Can you work these out from the model? Positions are in its coordinate system, mm. A direction names the side the tool comes from. Give positions to 0.01 mm unless a question says otherwise; leave off trailing zeros. Order: outer loops, then holes, each group sorted by start corner. A loop starts at its lowest first (then second) coordinate and runs counter-clockwise, first axis right, second up. Notation, with made-up numbers: (68, -11) - (103, -11) arc R8 ccw to (103, 2) - close; hole circle Ø8 at (48.5, 28). An arc over 180 degrees is marked (long way). Return JSON: item names as keys, results as strings.
```python
from build123d import *

# Parameters (mm, degrees)
SKETCH1_R           = 1.606483672
SKETCH1_R_2         = 1.474719506
BOSS_EXTRUDE1_DEPTH = 1
BOSS_EXTRUDE2_START = -2.5
SKETCH1_3_R         = 1.474719506
SKETCH1_3_R_2       = 1.606483672
BOSS_EXTRUDE2_DEPTH = 2.5


with BuildPart() as part:
    # Sketch1 → Boss-Extrude1 (new body)
    with BuildSketch(Plane(origin=(0, 0, 0), x_dir=(1, 0, 0), z_dir=(0, 1, 0))):
        with BuildLine():
            ThreePointArc((-516.919741048, 9.197616983), (-515.869047512, 9.418519621), (-514.947021866, 8.868407277))
            Line((-514.947021866, 8.868407277), (-509.711678857, 40.240087315))
            ThreePointArc((-509.711678857, 40.240087315), (-510.755516658, 40.060266208), (-511.684398038, 40.569297021))
            Line((-511.684398038, 40.569297021), (-516.919741048, 9.197616983))
        make_face()
        with Locations((-510.491081649, 41.644836785)):
            Circle(SKETCH1_R)
        with Locations((-516.1117935, 7.963915892)):
            Circle(SKETCH1_R_2)
    extrude(amount=BOSS_EXTRUDE1_DEPTH)

    # Sketch1_3 → Boss-Extrude2 (add)
    with BuildSketch(Plane(origin=(0, 0, 0), x_dir=(1, 0, 0), z_dir=(0, 1, 0)).offset(BOSS_EXTRUDE2_START)):
        with Locations(Location((-516.1117935, 7.963915892, 0), (0, 0, 123.220682047))):
            Circle(SKETCH1_3_R)
        with Locations(Location((-510.491081649, 41.644836785, 0), (0, 0, 222.028435657))):
            Circle(SKETCH1_3_R_2)
    extrude(amount=BOSS_EXTRUDE2_DEPTH)


solid = part.part
```
1. On a 3-axis mill with a long thin cutter (end or side, diameter ignored), from which of +Z, -Z, +X, -X, +Y, -Y can I reach the whole of each face in a straight line? I mean faces 4 (the face through (-510.199, -0.774, -43.224)), 5 (the face through (-510, -2.5, -42)). Say none if no direction works.
Checks:
{"face 4": "-Y", "face 5": "+Z, -Z, +X, -X, -Y"}
2. Suppose I cut it at C-C (z = -41). List the corners of the cut face in (x, y) for me.
Checks:
{"outline": "(-511.96, -2.5) - (-509.02, -2.5) - (-509.02, 1) - (-511.96, 1) - close"}
3. Thinking about a two-plate mould opening in Y: for faces 1 (the face through (-513, 1, -25)), 2 (the face through (-516, -2.5, -8)), 3 (the face through (-514.265, 0.493, -25.103)), which applies, +Y half, -Y half, draft (parallel to the pull), parting line (faces both ways), or undercut?
Checks:
{"face 1": "+Y half", "face 2": "-Y half", "face 3": "draft"}
4. Suppose I cut it at A-A (y = -1.8). List the corners of the cut face in (x, z) for me.
Checks:
{"outline": "circle Ø2.95 at (-516.11, -7.96); circle Ø3.21 at (-510.49, -41.64)"}
5. If I drill on L1, parallel to Y at x = -511.5, z = -39.5; L2, parallel to Z at x = -516, y = -1; L3, parallel to X at y = 0.3, z = -24, over which ranges is the centre line in solid material (lowest first)? Write a range as [from, to].
Checks:
{"L1": "[0, 1]", "L2": "[-9.43, -6.49]", "L3": "[-514.45, -512.42]"}
6. For pin 1 Ø5 at (x, z) = (-514, -29.5) entering from -Y; pin 2 Ø1.5 at (y, z) = (-2, -34.5) entering from +X, each with a flat end and sliding along its axis, tell me the tip position at first contact or that it passes through.
Checks:
{"pin 1": "y = 0", "pin 2": "through"}
7. Suppose I cut it at D-D (x = -510.25). List the corners of the cut face in (y, z) for me, plus the area to 3 significant figures.
Checks:
{"outline": "(-2.5, -43.23) - (1, -43.23) - (1, -37.01) - (0, -37.01) - (0, -40.06) - (-2.5, -40.06) - close", "area": "14.2 mm^2"}
8. Suppose I cut it at B-B (y = 0.65). List the corners of the cut face in (x, z) for me.
Checks:
{"outline": "(-516.92, -9.2) - (-511.68, -40.57) arc R1.61 ccw (long way) to (-509.71, -40.24) - (-514.95, -8.87) arc R1.47 ccw (long way) to start"}
